Geometry: final body of the model. Coordinates: model frame, mm. Face numbers are marked on the shaded views. A direction names the side the tool comes from. Give positions to 0.01 mm unless a question says otherwise; leave off trailing zeros. Write each loop counter-clockwise with the first axis right and the second up, starting at its lowest first coordinate (ties: lowest second). Pieces come first, ordered by that corner, then holes.
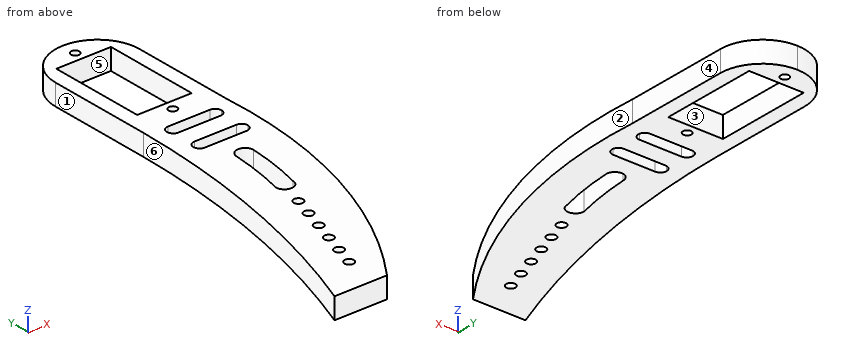
```python
from build123d import *

# Parameters (mm, degrees)
SKETCH1_W           = 20
SKETCH1_H           = 35
SKETCH1_W_2         = 13
SKETCH1_H_2         = 23
BOSS_EXTRUDE1_DEPTH = 5
SKETCH2_R           = 1
CUT_EXTRUDE1_DEPTH  = 5
BOSS_EXTRUDE2_DEPTH = 5
FILLET1_R           = 10
SKETCH6_R           = 1.1
CUT_EXTRUDE2_DEPTH  = 10
SKETCH7_W           = 13
SKETCH7_H           = 3
CUT_EXTRUDE3_DEPTH  = 10
FILLET2_R           = 1.5


with BuildPart() as part:
    # Sketch1 → Boss-Extrude1 (new body)
    with BuildSketch(Plane.XY):
        Rectangle(SKETCH1_W, SKETCH1_H)
        Rectangle(SKETCH1_W_2, SKETCH1_H_2, mode=Mode.SUBTRACT)
    extrude(amount=BOSS_EXTRUDE1_DEPTH)

    # Sketch2 → Cut-Extrude1 (cut)
    with BuildSketch(Plane.XY.offset(5)):
        with Locations((0, 13.9)):
            Circle(SKETCH2_R)
        with Locations(Location((0, -13.9, 0), (0, 0, 180))):
            Circle(SKETCH2_R)
    extrude(amount=-CUT_EXTRUDE1_DEPTH, mode=Mode.SUBTRACT)

    # Sketch4 → Boss-Extrude2 (add)
    with BuildSketch(Plane.XY.offset(5)):
        with BuildLine():
            Line((0, -17.5), (-10, -17.5))
            ThreePointArc((-10, -17.5), (-13.470780797, -53.21636341), (-23.268193188, -87.737598108))
            Line((-23.268193188, -87.737598108), (-10.768193188, -87.737598108))
            ThreePointArc((-10.768193188, -87.737598108), (5.633525229, -54.39811862), (10, -17.5))
            Line((10, -17.5), (0, -17.5))
        make_face()
    extrude(amount=-BOSS_EXTRUDE2_DEPTH)

    # Fillet1
    fillet1_edges = [part.edges().sort_by_distance(p)[0] for p in [
        (-10, 17.5, 2.5),
        (10, 17.5, 2.5),
    ]]
    fillet(fillet1_edges, radius=FILLET1_R - 0.0001)  # a hair under: the kernel refuses the full size

    # Sketch6 → Cut-Extrude2 (cut)
    with BuildSketch(Plane.XY.offset(5)):
        with Locations((-12.768649296, -79.368399131)):
            Circle(SKETCH6_R)
        with BuildLine():
            ThreePointArc((1.273336761, -35.373649828), (-0.726663239, -33.373649828), (-2.726663239, -35.373649828))
            ThreePointArc((-2.726663239, -35.373649828), (-3.473502661, -42.250603024), (-4.826684161, -49.034344928))
            ThreePointArc((-4.826684161, -49.034344928), (-2.826684161, -51.034344928), (-0.826684161, -49.034344928))
            ThreePointArc((-0.826684161, -49.034344928), (0.561306745, -42.255954178), (1.273336761, -35.373649828))
        make_face()
        with Locations((-11.211408841, -74.617083296)):
            Circle(SKETCH6_R)
        with Locations((-9.654168385, -69.865767461)):
            Circle(SKETCH6_R)
        with Locations((-8.09692793, -65.114451626)):
            Circle(SKETCH6_R)
        with Locations((-6.539687475, -60.363135791)):
            Circle(SKETCH6_R)
        with Locations((-4.98244702, -55.611819955)):
            Circle(SKETCH6_R)
    extrude(amount=-CUT_EXTRUDE2_DEPTH, mode=Mode.SUBTRACT)

    # Sketch7 → Cut-Extrude3 (cut)
    with BuildSketch(Plane.XY.offset(5)):
        with Locations((0, -27.5)):
            Rectangle(SKETCH7_W, SKETCH7_H)
        with Locations((0, -20)):
            Rectangle(SKETCH7_W, SKETCH7_H)
    extrude(amount=-CUT_EXTRUDE3_DEPTH, mode=Mode.SUBTRACT)

    # Fillet2
    fillet2_edges = [part.edges().sort_by_distance(p)[0] for p in [
        (6.5, -26, 2.5),
        (6.5, -29, 2.5),
        (-6.5, -29, 2.5),
        (-6.5, -26, 2.5),
        (6.5, -21.5, 2.5),
        (6.5, -18.5, 2.5),
        (-6.5, -21.5, 2.5),
        (-6.5, -18.5, 2.5),
    ]]
    fillet(fillet2_edges, radius=FILLET2_R - 0.0001)  # a hair under: the kernel refuses the full size


solid = part.part
```
Item 1: Section C-C, the plane y = 13.9. Return the cut outline in (x, z), plus the area to 3 significant figures.
Found:
outline: (-7.68, 0) - (-1, 0) - (-1, 5) - (-7.68, 5) - close; (1, 0) - (7.68, 0) - (7.68, 5) - (1, 5) - close
area: 66.8 mm2
Item 2: Section A-A, the plane y = -13.9. Return the cut outline in (x, z), plus the area to 3 significant figures.
Found:
outline: (-10, 0) - (-1, 0) - (-1, 5) - (-10, 5) - close; (1, 0) - (10, 0) - (10, 5) - (1, 5) - close
area: 90.0 mm2
Item 3: Pin query (flat end, axial travel): pin 1 Ø2 at (y, z) = (-20, 1.5) entering from -X; pin 2 Ø3 at (x, z) = (1, 4) entering from +Y; pin 3 Ø2.5 at (x, z) = (0, 3) entering from -Y; pin 4 Ø1.5 at (x, z) = (1, 3.5) entering from -Y. Return the tip coordinate at first contact, or that it passes through.
Found:
pin 1: stops at x = -10.06
pin 2: stops at y = 17.5
pin 3: stops at y = -71.97
pin 4: stops at y = -68.81
Item 4: Line query: L1, parallel to Y at x = 1.5, z = 1.25; L2, parallel to X at y = -9, z = 2.65; L3, parallel to Y at x = -5, z = 1.2. Output: solid intervals per line, ascending.
Found:
L1: y = -65.96 to -29, -26 to -21.5, -18.5 to -11.5, 11.5 to 17.39
L2: x = -10 to -6.5, 6.5 to 10
L3: y = -78.91 to -56.71, -54.51 to -29, -26 to -21.5, -18.5 to -11.5, 11.5 to 16.16
Item 5: Reachability of the marked faces 4, 5 and 6 from +Z, -Z, +X, -X, +Y, -Y: full face, straight path, thin tool, end or side. Return the list, or none.
Found:
face 4: +Z, -Z, +X, +Y
face 5: +Z, -Z
face 6: +Z, -Z, -X, +Y
Item 6: Pull-direction query (X, two-part tool) for the marked faces 1, 2 and 3; classes: +X half, -X half, draft (parallel to the pull), parting line (faces both ways), or undercut.
Found:
face 1: -X half
face 2: +X half
face 3: undercut
Item 7: Section B-B, the plane z = 1.65. State how many separate pieces and enclosed holes the cut face has, plus the area to 3 significant figures.
Found:
separate pieces: 1
enclosed holes: 12
area: 1,480 mm2
